```python
from build123d import *

# Parameters (mm, degrees)
F0_W     = 50.8
F0_H     = 6.35
F0_W_2   = 6.35
F0_H_2   = 50.8
F1_DEPTH = 6.35


with BuildPart() as f1:
    # F0 (on Front) → F1 (new body)
    with BuildSketch(Plane.XZ):
        Polygon((-69.85, 76.2), (-76.2, 76.2), (-76.2, 69.85), (-76.2, 19.05), (-76.2, -19.05), (-76.2, -69.85), (-76.2, -76.2), (-69.85, -76.2), (-19.05, -76.2), (19.05, -76.2), (69.85, -76.2), (76.2, -76.2), (76.2, -69.85), (76.2, -19.05), (76.2, 19.05), (76.2, 69.85), (76.2, 76.2), (69.85, 76.2), (19.05, 76.2), (-19.05, 76.2), align=None)
        with Locations((-44.45, 79.375)):
            Rectangle(F0_W, F0_H)
        with Locations((-79.375, 44.45)):
            Rectangle(F0_W_2, F0_H_2)
        with Locations((44.45, 79.375)):
            Rectangle(F0_W, F0_H)
        with Locations((-79.375, -44.45)):
            Rectangle(F0_W_2, F0_H_2)
        with Locations((79.375, 44.45)):
            Rectangle(F0_W_2, F0_H_2)
        with Locations((-44.45, -79.375)):
            Rectangle(F0_W, F0_H)
        with Locations((79.375, -44.45)):
            Rectangle(F0_W_2, F0_H_2)
        with Locations((44.45, -79.375)):
            Rectangle(F0_W, F0_H)
    extrude(amount=F1_DEPTH)


solid = f1.part
```
The listing builds one solid part. Answer for the finished solid, in the listing's coordinates (mm). A direction names the side the tool comes from. Give positions to 0.01 mm unless a question says otherwise; leave off trailing zeros. Order: outer loops, then holes, each group sorted by start corner. A loop starts at its lowest first (then second) coordinate and runs counter-clockwise, first axis right, second up.
Item 1: For a pull along Z with two mould halves and no side action, classify faces 6 (the face through (-79, -3, -19.05)), 7 (the face through (-73, -3, 76.2)), 8 (the face through (-76.2, -3, 73)) as pulls with the +Z half, pulls with the -Z half, needs draft (parallel to the pull), parting line crosses it, or undercut.
From the geometry:
face 6: undercut
face 7: pulls with the +Z half
face 8: needs draft
Item 2: Which of the six approach directions +Z, -Z, +X, -X, +Y, -Y give full straight-line access (tool end or side, diameter ignored) to faces 1 (the face through (-76.2, -3, 0)), 2 (the face through (69.85, -3, -79)), 3 (the face through (-19.05, -3, -79)), 4 (the face through (-79, -3, -69.85)), 5 (the face through (69.85, -3, 79))?
From the geometry:
face 1: -X, +Y, -Y
face 2: -Z, +X, +Y, -Y
face 3: -Z, +Y, -Y
face 4: -Z, -X, +Y, -Y
face 5: +Z, +X, +Y, -Y
Item 3: Find the intervals of material crossed by probe 1 along X at (y, z) = (-4.5, -8), in increasing order.
From the geometry:
probe 1: x = -76.2 to 76.2
Item 4: The part is cut by section B-B, the plane x = 8.5. Give the vertices of the cut face in (y, z), and give its area (3 significant figures).
From the geometry:
outline: (-6.35, -76.2) - (0, -76.2) - (0, 76.2) - (-6.35, 76.2) - close
area: 968 mm2
Item 5: The part is cut by section A-A, the plane z = -72. Give the vertices of the cut face in (x, y), and give its area (3 significant figures).
From the geometry:
outline: (-76.2, -6.35) - (76.2, -6.35) - (76.2, 0) - (-76.2, 0) - close
area: 968 mm2
Item 6: Given pin 1 Ø3 at (x, y) = (-74, -3) entering from -Z; pin 2 Ø3 at (y, z) = (-2.5, -78.5) entering from +X; pin 3 Ø6 at (x, z) = (-43.5, 23.5) entering from +Y; pin 4 Ø3 at (x, y) = (80.5, -2) entering from +Z, each flat-ended and moving along its own axis, determine where each tip first touches the part or whether it passes through.
From the geometry:
pin 1: stops at z = -76.2
pin 2: stops at x = 69.85
pin 3: stops at y = 0
pin 4: stops at z = 69.85
